Autodesk Inventor part; units mm, degrees
ref_plane "YZ Plane" through (0, 0, 0) normal (1, 0, 0) x (0, 1, 0)
ref_plane "XZ Plane" through (0, 0, 0) normal (0, 1, 0) x (-1, 0, 0)
ref_plane "XY Plane" through (0, 0, 0) normal (0, 0, 1) x (1, 0, 0)
sketch "Sketch1" plane through (0, 0, 0) normal (0, 0, 1) x (1, 0, 0)
  circle A0 centre (-12.936, 0.5481) radius 6.35
  circle A1 centre (-12.936, 0.5481) radius 14.1605
  point P0 (0, 0)
  dimension "d0" = 12.7
  dimension "d1" = 28.321
extrude "Extrusion1" add sketch "Sketch1" against normal blind 10.414
sketch "Sketch2" plane through (-12.936, 0.5481, -10.414) normal (0, 0, -1) x (-1, 0, 0)
  circle A0 centre (0, 0) radius 14.1605
  line L0 (3.1289, 6.6404) -> (-4.1863, 6.0299)
  line L1 (3.1289, 6.6404) -> (7.3152, 0.6105)
  line L2 (7.3152, 0.6105) -> (4.1863, -6.0299)
  line L3 (4.1863, -6.0299) -> (-3.1289, -6.6404)
  line L4 (-3.1289, -6.6404) -> (-7.3152, -0.6105)
  line L5 (-7.3152, -0.6105) -> (-4.1863, 6.0299)
  point P0 (-12.936, -0.5481)
  dimension "d5" = 7.3406
  dimension "d6" = 7.3406
  dimension "d7" = 7.3406
  dimension "d8" = 7.3406
  dimension "d9" = 120
  dimension "d10" = 120
  dimension "d11" = 120
  dimension "d12" = 7.3406
  dimension "d13" = 120
  dimension "d14" = 120
  dimension "d15" = 120
  dimension "d16" = 12.7143
  dimension "d17" = 6.3571
  dimension "d18" = 14.6303
  dimension "d19" = 7.3152
extrude "Extrusion2" cut sketch "Sketch2" against normal blind 25.4 contours L1 L2 L3 L4 L5 L0
equation "\"d6\" = d5"
equation "\"d7\" = d5"
equation "\"d8\" = d5"
equation "\"d9\" = d10"
equation "\"d12\" = d5"
equation "\"d17\" = 0.5 * d16"
equation "\"d19\" = 0.5 * d18"
properties part number "ShaftCollar"
Verification items for the finished model (mm, model axes). A direction names the side the tool comes from. Coordinates: 2 decimals unless noted, no trailing zeros. Order: outer loops, then holes, each group sorted by start corner. A loop starts at its lowest first (then second) coordinate and runs counter-clockwise, first axis right, second up.
1. Sectioned sample at D-D, the plane x = -23. Record the cut outline in (y, z).
Results found:
outline: (-9.41, -10.41) - (10.51, -10.41) - (10.51, 0) - (-9.41, 0) - close
2. Sectioned sample at C-C, the plane z = -1.75. Record the cut outline in (x, y), and give its area (3 significant figures).
Results found:
outline: circle Ø28.32 at (-12.94, 0.55); hole (-20.25, 1.16) - (-17.12, -5.48) - (-9.81, -6.09) - (-5.62, -0.06) - (-8.75, 6.58) - (-16.06, 7.19) - close
area: 490 mm2
3. Sectioned sample at B-B, the plane x = -14.5. Record the cut outline in (y, z), and give its area (3 significant figures).
Results found:
outline: (-13.53, -10.41) - (-5.7, -10.41) - (-5.7, 0) - (-13.53, 0) - close; (7.06, -10.41) - (14.62, -10.41) - (14.62, 0) - (7.06, 0) - close
area: 160 mm2
4. Release check for a two-part mould opening along Y. For faces 1 (the face through (-6.8, -2.4, 0)), 2 (the face through (-18.129, 4.216, -5.28)), 3 (the face through (-27.083, 1.171, -5.134)) record: +Y half, -Y half, draft (parallel to the pull), parting line (faces both ways), or undercut.
Results found:
face 1: draft
face 2: undercut
face 3: parting line
5. Sectioned sample at A-A, the plane y = 5.25. Record the cut outline in (x, z), and give its area (3 significant figures).
Results found:
outline: (-26.29, -10.41) - (-17.41, -10.41) - (-17.41, 0) - (-26.29, 0) - close; (-8.12, -10.41) - (0.42, -10.41) - (0.42, 0) - (-8.12, 0) - close
area: 181 mm2
6. Set-up check for faces 4 (the face through (-6.8, -2.4, -10.414)), 5 (the face through (-7.743, -3.12, -5.28)): record each of +Z, -Z, +X, -X, +Y, -Y from which the full face is reachable in a straight line by a thin tool's end or side.
Results found:
face 4: -Z, +X, -X, +Y, -Y
face 5: +Z, -Z
7. Scan lines: line 1 (Y direction, x = -17.25, z = -4.75); line 2 (Y direction, x = -14.25, z = -7.25); line 3 (X direction, y = 0.75, z = -3.75). Record each from-to range of solid material in increasing order.
Results found:
line 1: y = -12.94 to -5.21, 5.48 to 14.04
line 2: y = -13.55 to -5.72, 7.04 to 14.65
line 3: x = -27.1 to -20.06, -6 to 1.22
8. Go/stop test with flat-tipped pins: pin 1 Ø1.5 at (x, z) = (-17, -3.5) entering from +Y; pin 2 Ø6 at (x, z) = (-20.5, -3.5) entering from +Y; pin 3 Ø2 at (x, z) = (-10, -3.5) entering from +Y. Record where each tip stops, or that it passes through.
Results found:
pin 1: stops at y = 14.32
pin 2: stops at y = 13.95
pin 3: stops at y = 14.58
